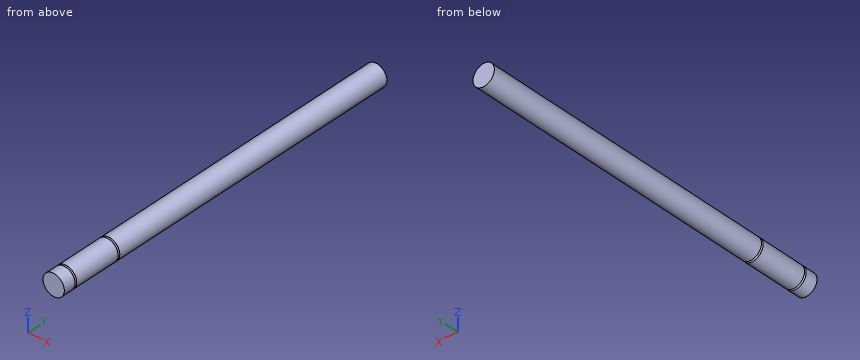
from build123d import *

# Parameters (mm, degrees)
SKETCH1_R           = 4
BOSS_EXTRUDE1_DEPTH = 135
SKETCH2_W           = 1
SKETCH2_H           = 0.7
LPATTERN1_COUNT     = 2
LPATTERN1_PITCH     = 18


with BuildPart() as part:
    # Sketch1 → Boss-Extrude1 (new body)
    with BuildSketch(Plane(origin=(0, 0, 0), x_dir=(1, 0, 0), z_dir=(0, 1, 0))):
        with Locations(Location((0, 0, 0), (0, 0, 270))):
            Circle(SKETCH1_R)
    extrude(amount=BOSS_EXTRUDE1_DEPTH)

    # Sketch2 → Cut-Revolve1 (revolve, cut)
    with BuildSketch(Plane.XY, mode=Mode.PRIVATE) as cut_revolve1_sk:
        with Locations((-3.5, 4.85)):
            Rectangle(SKETCH2_W, SKETCH2_H)
    cut_revolve1 = revolve(cut_revolve1_sk.sketch.rotate(Axis((0, 0, 0), (0, 1, 0)), 270), axis=Axis((0, 0, 0), (0, 1, 0)), mode=Mode.SUBTRACT)

    # LPattern1: Cut-Revolve1 ×2
    with Locations(*[(0, i * LPATTERN1_PITCH, 0) for i in range(1, LPATTERN1_COUNT)]):
        add(cut_revolve1, mode=Mode.SUBTRACT)


solid = part.part
Source: CAD feature listing. Evaluate the final solid. Frame: model axes, mm. Coordinates: 2 decimals unless noted, no trailing zeros. Write each loop counter-clockwise with the first axis right and the second up, starting at its lowest first coordinate (ties: lowest second). Pieces come first, ordered by that corner, then holes. Notation, with made-up numbers: M -27.75,66 L 9.25,66 A26 cw 9.25,94 Z; hole C 82,46 d11. An arc over 180 degrees is marked long. Use a Markdown table: item, result.
1) First-contact query: pin 1 Ø2 at (y, z) = (99, -1) entering from +X; pin 2 Ø2 at (y, z) = (73, -2) entering from +X. Flat tips, straight axial feed; report the tip coordinate or a pass-through.
Conclusion:
| item | result |
|---|---|
| pin 1 | stops at x = 4 |
| pin 2 | stops at x = 3.87 |
2) Section B-B, the plane x = -1.5. Output: boundary loops of the cut face in (y, z).
Conclusion:
| item | result |
|---|---|
| outline | M 0,-3.71 L 4.5,-3.71 L 4.5,-2.6 L 5.2,-2.6 L 5.2,-3.71 L 22.5,-3.71 L 22.5,-2.6 L 23.2,-2.6 L 23.2,-3.71 L 135,-3.71 L 135,3.71 L 23.2,3.71 L 23.2,2.6 L 22.5,2.6 L 22.5,3.71 L 5.2,3.71 L 5.2,2.6 L 4.5,2.6 L 4.5,3.71 L 0,3.71 Z |
3) Ray query, L1, parallel to Y at x = -2.25, z = -2.75; L2, parallel to Z at x = 0.25, y = 97.5. Return the intervals inside material, ascending.
Conclusion:
| item | result |
|---|---|
| L1 | y = 0 to 4.5, 5.2 to 22.5, 23.2 to 135 |
| L2 | z = -3.99 to 3.99 |
4) Section C-C, the plane y = 125. Output: boundary loops of the cut face in (x, z).
Conclusion:
| item | result |
|---|---|
| outline | C 0,0 d8 |
5) Section A-A, the plane z = 0.75. Output: boundary loops of the cut face in (x, y), then the cut area to 3 significant figures.
Conclusion:
| item | result |
|---|---|
| outline | M -3.93,0 L 3.93,0 L 3.93,4.5 L 2.9,4.5 L 2.9,5.2 L 3.93,5.2 L 3.93,22.5 L 2.9,22.5 L 2.9,23.2 L 3.93,23.2 L 3.93,135 L -3.93,135 L -3.93,23.2 L -2.9,23.2 L -2.9,22.5 L -3.93,22.5 L -3.93,5.2 L -2.9,5.2 L -2.9,4.5 L -3.93,4.5 Z |
| area | 1,060 mm^2 |
